Geometry: final body of the model. Coordinates: model frame, mm. A direction names the side the tool comes from. Give positions to 0.01 mm unless a question says otherwise; leave off trailing zeros. Write each loop counter-clockwise with the first axis right and the second up, starting at its lowest first coordinate (ties: lowest second). Pieces come first, ordered by that corner, then holes. Notation, with made-up numbers: M 17.5,-9.75 L 39.5,-9.75 A26 cw 39.5,9.25 Z; hole C 18.25,79 d1. An arc over 180 degrees is marked long. Answer as a JSON object with one key per item and string values.
from build123d import *

# Parameters (mm, degrees)
KES_EKSTR_ZYON1_DEPTH = 1


with BuildPart() as part:
    # Çizim1 → Döndür1 (revolve)
    with BuildSketch(Plane.XY, mode=Mode.PRIVATE) as d_nd_r1_sk:
        with BuildLine():
            Line((-17.895152368, 0), (-17.895152368, 1.425))
            ThreePointArc((-17.895152368, 1.425), (-17.521324038, 2.389446085), (-16.595152368, 2.85))
            Line((-16.595152368, 2.85), (-16.245152368, 2.85))
            Line((-16.245152368, 2.85), (-16.245152368, 1.5))
            Line((-16.245152368, 1.5), (20.454847632, 1.5))
            Line((20.454847632, 1.5), (20.754847632, 1.2))
            Line((20.754847632, 1.2), (20.754847632, 0))
            Line((20.754847632, 0), (-17.895152368, 0))
        make_face()
    revolve(d_nd_r1_sk.sketch.rotate(Axis((-8.74874301, 0, 0), (1, 0, 0)), 90), axis=Axis((-8.74874301, 0, 0), (1, 0, 0)))

    # Çizim2 → Kes-Ekstrüzyon1 (cut)
    with BuildSketch(Plane.ZY.offset(17.895152368)):
        Polygon((0, 1.154700538), (-1, 0.577350269), (-1, -0.577350269), (0, -1.154700538), (1, -0.577350269), (1, 0.577350269), align=None)
    extrude(amount=-KES_EKSTR_ZYON1_DEPTH, mode=Mode.SUBTRACT)


solid = part.part
1) Contact query for flat-ended pins moving along their axis: P1, Ø0.8, axis at x = -17.5, y = 0, coming from the +Z side; P2, Ø1, axis at x = -9, z = 1, coming from the +Y side; P3, Ø1.5, axis at x = 6, z = 2, coming from the -Y side. Output: stop coordinate, or through.
Geometry check:
{"P1": "stops at z = 2.71", "P2": "stops at y = 1.41", "P3": "stops at y = -0.83"}
2) Line query: line 1 (Y direction, x = 11, z = 0); line 2 (Y direction, x = 8, z = 0.95); line 3 (X direction, y = 1.65, z = 0.3). Output: solid intervals per line, ascending. Write a range as from..to.
Geometry check:
{"line 1": "y = -1.5..1.5", "line 2": "y = -1.16..1.16", "line 3": "x = -17.87..-16.25"}
3) Pull-direction query (Y, two-part tool) for faces 3 (the flat face through (-17.4, 0, 1)), 4 (the flat face through (-16.245, 1.2, 1.2)), 5 (the flat face through (-17.4, 0, -1)), 6 (the cylindrical face through (2.36, -0.45, 1.43)); classes: pulls with the +Y half, pulls with the -Y half, needs draft (parallel to the pull), parting line crosses it, or undercut.
Geometry check:
{"face 3": "undercut", "face 4": "needs draft", "face 5": "undercut", "face 6": "parting line crosses it"}
4) Set-up query: faces 1 (the flat face through (20.755, 0, 0)), 2 (the flat face through (-17.4, 0.87, -0.49)). Return all of +Z, -Z, +X, -X, +Y, -Y with unobstructed straight access to the full face (end or side cutting, diameter ignored); none if empty.
Geometry check:
{"face 1": "+Z, -Z, +X, +Y, -Y", "face 2": "-X"}
5) Cut plane A-A on x = 8. Return loops of the section in (y, z).
Geometry check:
{"outline": "C 0,0 d3"}
